Source: three-view drawing plus pictorial views. Frame: mm from the lowest corner of the part. Coordinates: 2 decimals unless noted, no trailing zeros. Write each loop counter-clockwise with the first axis right and the second up, starting at its lowest first coordinate (ties: lowest second). Pieces come first, ordered by that corner, then holes. Notation, with made-up numbers: (83.5, 71) - (139.5, 71) arc R18 ccw to (139.5, 85) - close; hole circle Ø1 at (71, 60). An arc over 180 degrees is marked (long way). Put each result on its own line as item: value. Start each with the question number.
1. Cut plane A-A, the plane x = 6. Return loops of the section in (y, z), and give its area (3 significant figures).
2. Pull-direction query (Z, two-part tool) for the marked faces 1, 2 and 3; classes: released by +Z, released by -Z, zero draft, split by the parting line, or undercut.
3. Line query: line 1 (Y direction, x = 61, z = 11); line 2 (X direction, y = 6.5, z = 3.5); line 3 (X direction, y = 11, z = 11.5). Output: solid intervals per line, ascending.
4. Cut plane D-D, the plane y = 3.25. Return loops of the section in (x, z).
5. Cut plane B-B, the plane z = 6.75. Return loops of the section in (x, y), and give its area (3 significant figures).
6. Cut plane C-C, the plane y = 6.75. Return loops of the section in (x, z).
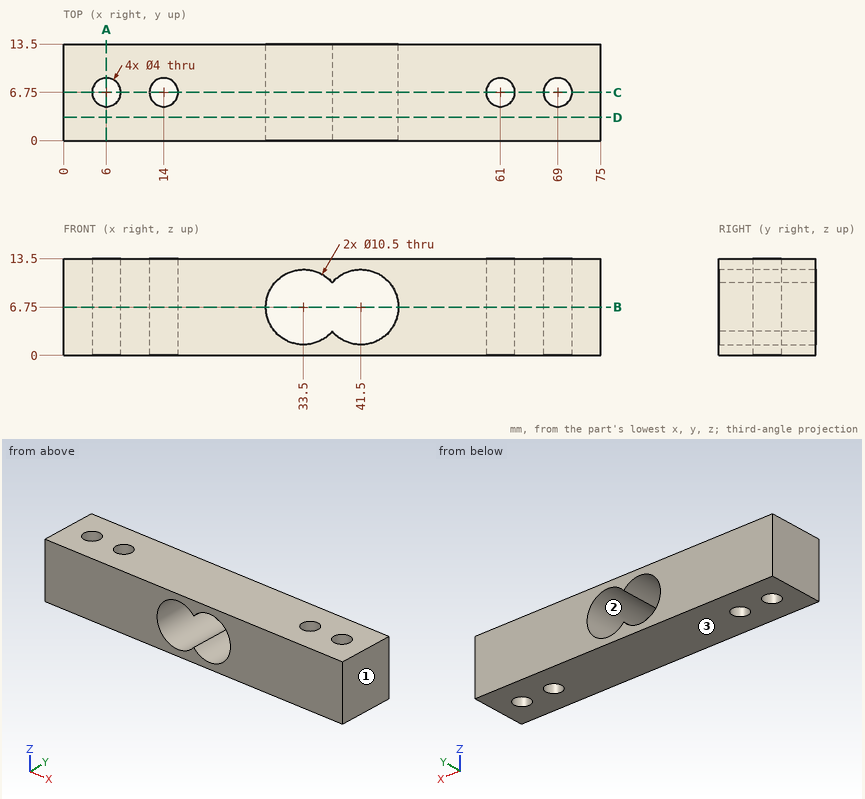
Report:
1. outline: (0, 0) - (4.75, 0) - (4.75, 13.5) - (0, 13.5) - close; (8.75, 0) - (13.5, 0) - (13.5, 13.5) - (8.75, 13.5) - close
1. area: 128 mm^2
2. face 1: zero draft
2. face 2: undercut
2. face 3: released by -Z
3. line 1: y = 0 to 4.75, 8.75 to 13.5
3. line 2: x = 0 to 4.02, 7.98 to 12.02, 15.98 to 29.38, 45.62 to 59.02, 62.98 to 67.02, 70.98 to 75
3. line 3: x = 0 to 31.26, 35.74 to 39.26, 43.74 to 75
4. outline: (0, 0) - (75, 0) - (75, 13.5) - (0, 13.5) - close; hole (37.5, 3.35) arc R5.25 ccw (long way) to (37.5, 10.15) arc R5.25 ccw (long way) to start
5. outline: (0, 0) - (28.25, 0) - (28.25, 13.5) - (0, 13.5) - close; (46.75, 0) - (75, 0) - (75, 13.5) - (46.75, 13.5) - close; hole circle Ø4 at (6, 6.75); hole circle Ø4 at (14, 6.75); hole circle Ø4 at (61, 6.75); hole circle Ø4 at (69, 6.75)
5. area: 712 mm^2
6. outline: (0, 0) - (4, 0) - (4, 13.5) - (0, 13.5) - close; (8, 0) - (12, 0) - (12, 13.5) - (8, 13.5) - close; (16, 0) - (59, 0) - (59, 13.5) - (16, 13.5) - close; (63, 0) - (67, 0) - (67, 13.5) - (63, 13.5) - close; (71, 0) - (75, 0) - (75, 13.5) - (71, 13.5) - close; hole (37.5, 3.35) arc R5.25 ccw (long way) to (37.5, 10.15) arc R5.25 ccw (long way) to start
